Autodesk Inventor part; units mm, degrees
ref_plane "YZ Plane" through (0, 0, 0) normal (1, 0, 0) x (0, 1, 0)
ref_plane "XZ Plane" through (0, 0, 0) normal (0, 1, 0) x (-1, 0, 0)
ref_plane "XY Plane" through (0, 0, 0) normal (0, 0, 1) x (1, 0, 0)
sketch "Esboço1" plane through (0, 0, 0) normal (0, 1, 0) x (-1, 0, 0)
  line L0 (-51.5, 51.5) -> (51.5, 51.5)
  line L1 (51.5, 51.5) -> (51.5, -51.5)
  line L2 (51.5, -51.5) -> (-51.5, -51.5)
  line L3 (-51.5, -51.5) -> (-51.5, 51.5)
  line L4 (-51.5, 51.5) -> (51.5, -51.5) construction
  line L5 (51.5, 51.5) -> (-51.5, -51.5) construction
  point P0 (0, 0)
  dimension "d0" = 103
  dimension "d1" = 103
extrude "Extrusão1" add sketch "Esboço1" along normal blind 40
sketch "Esboço2" plane through (0, 40, 0) normal (0, 1, 0) x (1, 0, 0)
  line L0 (51.5, 51.5) -> (-51.5, 51.5)
  line L1 (-51.5, 51.5) -> (-51.5, -51.5)
  line L2 (-51.5, -51.5) -> (51.5, -51.5)
  line L3 (51.5, -51.5) -> (51.5, 51.5)
  line L4 (-50, -50) -> (-50, 50)
  line L5 (-50, 50) -> (50, 50)
  line L6 (50, 50) -> (50, -50)
  line L7 (50, -50) -> (-50, -50)
  point P0 (0, 0)
  dimension "d4" = 1.5
extrude "Extrusão2" cut sketch "Esboço2" against normal blind 38.5 contours L4 L5 L6 L7
properties part number "Gabarito" material "Madeira (Cerejeira)"
Verification items for the finished model (mm, model axes). A direction names the side the tool comes from. Give positions to 0.01 mm unless a question says otherwise; leave off trailing zeros. Loops run counter-clockwise (first coordinate to the right, second up) from the corner with the lowest first, then second, coordinate; pieces in that order, holes last. Notation, with made-up numbers: M 85.25,-20 L 133.25,-20 A26 cw 133.25,-1 Z; hole C 1,51 d6. An arc over 180 degrees is marked long. Return JSON: item names as keys, results as strings.
1) Section check B-B, the plane z = 18. Enter the section's corners in (x, y).
Findings:
{"outline": "M -51.5,0 L 51.5,0 L 51.5,40 L 50,40 L 50,1.5 L -50,1.5 L -50,40 L -51.5,40 Z"}
2) Section check A-A, the plane y = 30. Enter the section's corners in (x, z), and give its area (3 significant figures).
Findings:
{"outline": "M -51.5,-51.5 L 51.5,-51.5 L 51.5,51.5 L -51.5,51.5 Z; hole M -50,-50 L 50,-50 L 50,50 L -50,50 Z", "area": "609 mm2"}
3) Material ranges on L1, parallel to Z at x = 37.5, y = 20; L2, parallel to Y at x = 38, z = -21, recorded low to high. Write a range as [from, to].
Findings:
{"L1": "z = [-51.5, -50], [50, 51.5]", "L2": "y = [0, 1.5]"}
4) Tool access check on faces 5 (the flat face through (-1, 20, -51.5)), 6 (the flat face through (-1, 21, -50)). Record the directions out of +Z, -Z, +X, -X, +Y, -Y that give a thin tool (end or side, any length) a straight path to the whole face; none if there is none.
Findings:
{"face 5": "-Z, +X, -X, +Y, -Y", "face 6": "+Y"}
5) Gauge pin test, flat end, axial feed: P1, Ø2, axis at x = -32.5, z = -34, coming from the +Y side. Record the tip position at first contact, or that the pin passes through.
Findings:
{"P1": "stops at y = 1.5"}
6) Mould release check, pull along X, two halves, no side actions. Record for faces 1 (the flat face through (51.5, 20, -1)), 2 (the flat face through (1, 0, 1)), 3 (the flat face through (-50, 21, 1)), 4 (the flat face through (-1, 1.5, -1)): released by +X, released by -X, zero draft, split by the parting line, or undercut.
Findings:
{"face 1": "released by +X", "face 2": "zero draft", "face 3": "undercut", "face 4": "undercut"}
7) Section check C-C, the plane x = -0.5. Enter the section's corners in (y, z).
Findings:
{"outline": "M 0,-51.5 L 40,-51.5 L 40,-50 L 1.5,-50 L 1.5,50 L 40,50 L 40,51.5 L 0,51.5 Z"}
